from build123d import *

# Parameters (mm, degrees)
SKETCH1_R           = 4.9
SKETCH1_R_2         = 1.7
BOSS_EXTRUDE1_DEPTH = 19.8
SKETCH2_R           = 2.2
SKETCH2_R_2         = 1.7
BOSS_EXTRUDE2_DEPTH = 1.5
CHAMFER1_SIZE       = 0.25


with BuildPart() as part:
    # Sketch1 → Boss-Extrude1 (new body)
    with BuildSketch(Plane.XY):
        with Locations(Location((0, 0, 0), (0, 0, 180))):
            Circle(SKETCH1_R)
        with Locations(Location((0, 0, 0), (0, 0, 180))):
            Circle(SKETCH1_R_2, mode=Mode.SUBTRACT)
    extrude(amount=BOSS_EXTRUDE1_DEPTH)

    # Sketch2 → Boss-Extrude2 (add)
    with BuildSketch(Plane.XY.offset(19.8)):
        Circle(SKETCH2_R)
        with Locations(Location((0, 0, 0), (0, 0, 180))):
            Circle(SKETCH2_R_2, mode=Mode.SUBTRACT)
    extrude(amount=BOSS_EXTRUDE2_DEPTH)

    # Chamfer1
    chamfer1_edges = [part.edges().sort_by_distance(p)[0] for p in [
        (4.9, 0, 0),
        (1.7, 0, 0),
    ]]
    chamfer(chamfer1_edges, length=CHAMFER1_SIZE)


solid = part.part
The listing builds one solid part. Answer for the finished solid, in the listing's coordinates (mm). A direction names the side the tool comes from. Round coordinates to 2 decimals unless told otherwise and drop trailing zeros. Write each loop counter-clockwise with the first axis right and the second up, starting at its lowest first coordinate (ties: lowest second). Pieces come first, ordered by that corner, then holes. Notation, with made-up numbers: M 38,36.25 L 43,36.25 A13 cw 43,44.25 Z; hole C 56,5.25 d2. An arc over 180 degrees is marked long. Write each question's results on one line, items separated by ' | '. Start each with the question number.
Item 1: Flat-ended cylindrical pins translate along their axes: pin 1 Ø3 at (x, z) = (-3.5, 10) entering from +Y; pin 2 Ø1 at (x, y) = (-0.5, 0) entering from +Z. Find the tip coordinate at first contact, or state that the pin passes through.
Item 2: Straight lines are drawn through the part: L1, parallel to Y at x = 0, z = 12.25; L2, parallel to Z at x = 3.25, y = -0.5; L3, parallel to X at y = 1.5, z = 5. For each, find the intervals that lie inside material, in ascending order. Write a range as [from, to].
Item 3: For a pull along X with two mould halves and no side action, classify faces 3 (the face through (-2, 1, 0)), 4 (the face through (0.37, 1.66, 10.63)), 5 (the face through (3.612, -3.312, 9.888)) as pulls with the +X half, pulls with the -X half, needs draft (parallel to the pull), parting line crosses it, or undercut.
Item 4: For faces 1 (the face through (-2, 0, 21.3)), 2 (the face through (-2.1, -1.2, 19.8)), determine the directions among +Z, -Z, +X, -X, +Y, -Y from which every point of the face is accessible in a straight line to the end or side of a thin tool.
Item 5: A cutting plane is placed at A-A on x = 0. Write down the section's boundary in (y, z).
Item 6: A cutting plane is placed at C-C on z = 16.25. Write down the section's boundary in (x, y).
Check sheet entries:
1) pin 1: y = 4.47 | pin 2: through
2) L1: [-4.9, -1.7], [1.7, 4.9] | L2: [0, 19.8] | L3: [-4.66, -0.8], [0.8, 4.66]
3) face 3: needs draft | face 4: undercut | face 5: parting line crosses it
4) face 1: +Z, +X, -X, +Y, -Y | face 2: +Z
5) outline: M -4.9,0.25 L -4.65,0 L -1.95,0 L -1.7,0.25 L -1.7,21.3 L -2.2,21.3 L -2.2,19.8 L -4.9,19.8 Z; M 1.7,0.25 L 1.95,0 L 4.65,0 L 4.9,0.25 L 4.9,19.8 L 2.2,19.8 L 2.2,21.3 L 1.7,21.3 Z
6) outline: C 0,0 d9.8; hole C 0,0 d3.4
